Geometry check sheet. Reference: the model listing, model coordinates, mm. Face numbers are marked on the shaded views. A direction names the side the tool comes from. Give positions to 0.01 mm unless a question says otherwise; leave off trailing zeros. Loops run counter-clockwise (first coordinate to the right, second up) from the corner with the lowest first, then second, coordinate; pieces in that order, holes last. Notation, with made-up numbers: (41, -38) - (53, -38) arc R29 cw to (53, -17) - close; hole circle Ø8 at (6.25, -12.5). An arc over 180 degrees is marked (long way). Use a Markdown table: item, result. Add a question column.
1. Draft check along Z on the marked faces 3, 4, 5 and 6. Enter one of: pulls with the +Z half, pulls with the -Z half, needs draft (parallel to the pull), parting line crosses it, or undercut.
2. Cross-section at B-B on z = -15. Enter the section's corners in (x, y), and give its area (4 significant figures).
3. Set-up check for the marked faces 1 and 2: record each of +Z, -Z, +X, -X, +Y, -Y from which the full face is reachable in a straight line by a thin tool's end or side.
4. Material ranges on L1, parallel to Z at x = 25.5, y = 1; L2, parallel to Z at x = 101, y = 2.75; L3, parallel to Y at x = 8.5, z = -17.75, recorded low to high.
5. Depth check by flat-ended pin: P1, Ø2.5, axis at y = 3.5, z = -19, coming from the -X side. Enter the tip coordinate at first touch or a pass-through.
6. Cross-section at A-A on x = 101. Enter the section's corners in (y, z), and give its area (3 significant figures).
7. Cross-section at C-C on z = -6.25. Count the separate pieces of the cut face and the enclosed holes in it, and give its area (3 significant figures).
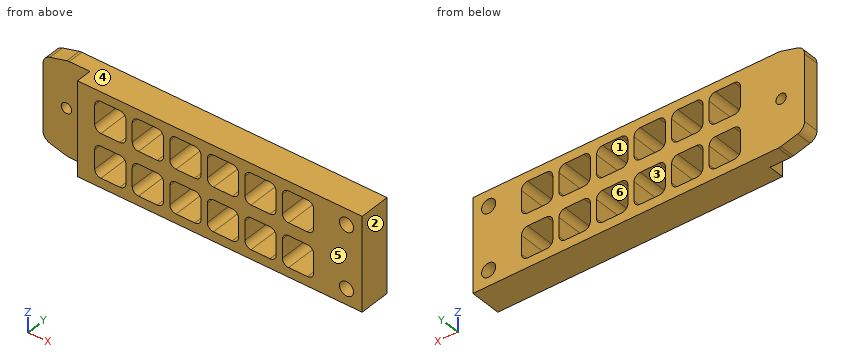
from build123d import *

# Parameters (mm, degrees)
EXTRUDE_1_DEPTH     = 10
SKETCH_4_W          = 15
SKETCH_4_H          = 30
CUT_EXTRUDE_2_DEPTH = 5
FILLET_1_R          = 3
CUT_EXTRUDE_3_DEPTH = 111.616454472
HOLE_WIZARD_M41_D   = 4.5
M4X0_71_D           = 3.3


with BuildPart() as part:
    # Эскиз1 → Бобышка-Вытянуть1 (new body)
    with BuildSketch(Plane(origin=(0, 0, 0), x_dir=(1, 0, 0), z_dir=(0, 1, 0))):
        Polygon((15, 0), (106, 0), (106, 30), (15, 30), (8, 30), (0, 27.856406461), (0, 2.143593539), (8, 0), align=None)
    extrude(amount=EXTRUDE_1_DEPTH)

    # Эскиз4 → Вырез-Вытянуть2 (cut)
    with BuildSketch(Plane.XZ):
        with Locations((7.5, -15)):
            Rectangle(SKETCH_4_W, SKETCH_4_H)
    extrude(amount=-CUT_EXTRUDE_2_DEPTH, mode=Mode.SUBTRACT)

    # Скругление1
    fillet_1_edges = [part.edges().sort_by_distance(p)[0] for p in [
        (8, 7.5, 0),
        (0, 7.5, -2.143593539),
        (0, 7.5, -27.856406461),
        (8, 7.5, -30),
    ]]
    fillet(fillet_1_edges, radius=FILLET_1_R)

    # Эскиз5 → Вырез-Вытянуть3 (cut, through all)
    with BuildSketch(Plane.XZ):
        with BuildLine():
            Line((22.5, -17), (28.5, -17))
            ThreePointArc((28.5, -17), (29.914213562, -17.585786438), (30.5, -19))
            Line((30.5, -19), (30.5, -25))
            ThreePointArc((30.5, -25), (29.914213562, -26.414213562), (28.5, -27))
            Line((28.5, -27), (22.5, -27))
            ThreePointArc((22.5, -27), (21.085786438, -26.414213562), (20.5, -25))
            Line((20.5, -25), (20.5, -19))
            ThreePointArc((20.5, -19), (21.085786438, -17.585786438), (22.5, -17))
        make_face()
        with BuildLine():
            Line((34.5, -17), (40.5, -17))
            ThreePointArc((40.5, -17), (41.914213562, -17.585786438), (42.5, -19))
            Line((42.5, -19), (42.5, -25))
            ThreePointArc((42.5, -25), (41.914213562, -26.414213562), (40.5, -27))
            Line((40.5, -27), (34.5, -27))
            ThreePointArc((34.5, -27), (33.085786438, -26.414213562), (32.5, -25))
            Line((32.5, -25), (32.5, -19))
            ThreePointArc((32.5, -19), (33.085786438, -17.585786438), (34.5, -17))
        make_face()
        with BuildLine():
            Line((46.5, -17), (52.5, -17))
            ThreePointArc((52.5, -17), (53.914213562, -17.585786438), (54.5, -19))
            Line((54.5, -19), (54.5, -25))
            ThreePointArc((54.5, -25), (53.914213562, -26.414213562), (52.5, -27))
            Line((52.5, -27), (46.5, -27))
            ThreePointArc((46.5, -27), (45.085786438, -26.414213562), (44.5, -25))
            Line((44.5, -25), (44.5, -19))
            ThreePointArc((44.5, -19), (45.085786438, -17.585786438), (46.5, -17))
        make_face()
        with BuildLine():
            Line((58.5, -17), (64.5, -17))
            ThreePointArc((64.5, -17), (65.914213562, -17.585786438), (66.5, -19))
            Line((66.5, -19), (66.5, -25))
            ThreePointArc((66.5, -25), (65.914213562, -26.414213562), (64.5, -27))
            Line((64.5, -27), (58.5, -27))
            ThreePointArc((58.5, -27), (57.085786438, -26.414213562), (56.5, -25))
            Line((56.5, -25), (56.5, -19))
            ThreePointArc((56.5, -19), (57.085786438, -17.585786438), (58.5, -17))
        make_face()
        with BuildLine():
            Line((70.5, -17), (76.5, -17))
            ThreePointArc((76.5, -17), (77.914213562, -17.585786438), (78.5, -19))
            Line((78.5, -19), (78.5, -25))
            ThreePointArc((78.5, -25), (77.914213562, -26.414213562), (76.5, -27))
            Line((76.5, -27), (70.5, -27))
            ThreePointArc((70.5, -27), (69.085786438, -26.414213562), (68.5, -25))
            Line((68.5, -25), (68.5, -19))
            ThreePointArc((68.5, -19), (69.085786438, -17.585786438), (70.5, -17))
        make_face()
        with BuildLine():
            Line((82.5, -17), (88.5, -17))
            ThreePointArc((88.5, -17), (89.914213562, -17.585786438), (90.5, -19))
            Line((90.5, -19), (90.5, -25))
            ThreePointArc((90.5, -25), (89.914213562, -26.414213562), (88.5, -27))
            Line((88.5, -27), (82.5, -27))
            ThreePointArc((82.5, -27), (81.085786438, -26.414213562), (80.5, -25))
            Line((80.5, -25), (80.5, -19))
            ThreePointArc((80.5, -19), (81.085786438, -17.585786438), (82.5, -17))
        make_face()
        with BuildLine():
            Line((90.5, -11), (90.5, -5))
            ThreePointArc((90.5, -5), (89.914213562, -3.585786438), (88.5, -3))
            Line((88.5, -3), (82.5, -3))
            ThreePointArc((82.5, -3), (81.085786438, -3.585786438), (80.5, -5))
            Line((80.5, -5), (80.5, -11))
            ThreePointArc((80.5, -11), (81.085786438, -12.414213562), (82.5, -13))
            Line((82.5, -13), (88.5, -13))
            ThreePointArc((88.5, -13), (89.914213562, -12.414213562), (90.5, -11))
        make_face()
        with BuildLine():
            Line((78.5, -11), (78.5, -5))
            ThreePointArc((78.5, -5), (77.914213562, -3.585786438), (76.5, -3))
            Line((76.5, -3), (70.5, -3))
            ThreePointArc((70.5, -3), (69.085786438, -3.585786438), (68.5, -5))
            Line((68.5, -5), (68.5, -11))
            ThreePointArc((68.5, -11), (69.085786438, -12.414213562), (70.5, -13))
            Line((70.5, -13), (76.5, -13))
            ThreePointArc((76.5, -13), (77.914213562, -12.414213562), (78.5, -11))
        make_face()
        with BuildLine():
            Line((66.5, -11), (66.5, -5))
            ThreePointArc((66.5, -5), (65.914213562, -3.585786438), (64.5, -3))
            Line((64.5, -3), (58.5, -3))
            ThreePointArc((58.5, -3), (57.085786438, -3.585786438), (56.5, -5))
            Line((56.5, -5), (56.5, -11))
            ThreePointArc((56.5, -11), (57.085786438, -12.414213562), (58.5, -13))
            Line((58.5, -13), (64.5, -13))
            ThreePointArc((64.5, -13), (65.914213562, -12.414213562), (66.5, -11))
        make_face()
        with BuildLine():
            Line((54.5, -11), (54.5, -5))
            ThreePointArc((54.5, -5), (53.914213562, -3.585786438), (52.5, -3))
            Line((52.5, -3), (46.5, -3))
            ThreePointArc((46.5, -3), (45.085786438, -3.585786438), (44.5, -5))
            Line((44.5, -5), (44.5, -11))
            ThreePointArc((44.5, -11), (45.085786438, -12.414213562), (46.5, -13))
            Line((46.5, -13), (52.5, -13))
            ThreePointArc((52.5, -13), (53.914213562, -12.414213562), (54.5, -11))
        make_face()
        with BuildLine():
            Line((42.5, -11), (42.5, -5))
            ThreePointArc((42.5, -5), (41.914213562, -3.585786438), (40.5, -3))
            Line((40.5, -3), (34.5, -3))
            ThreePointArc((34.5, -3), (33.085786438, -3.585786438), (32.5, -5))
            Line((32.5, -5), (32.5, -11))
            ThreePointArc((32.5, -11), (33.085786438, -12.414213562), (34.5, -13))
            Line((34.5, -13), (40.5, -13))
            ThreePointArc((40.5, -13), (41.914213562, -12.414213562), (42.5, -11))
        make_face()
        with BuildLine():
            Line((30.5, -11), (30.5, -5))
            ThreePointArc((30.5, -5), (29.914213562, -3.585786438), (28.5, -3))
            Line((28.5, -3), (22.5, -3))
            ThreePointArc((22.5, -3), (21.085786438, -3.585786438), (20.5, -5))
            Line((20.5, -5), (20.5, -11))
            ThreePointArc((20.5, -11), (21.085786438, -12.414213562), (22.5, -13))
            Line((22.5, -13), (28.5, -13))
            ThreePointArc((28.5, -13), (29.914213562, -12.414213562), (30.5, -11))
        make_face()
    extrude(amount=-CUT_EXTRUDE_3_DEPTH, mode=Mode.SUBTRACT)

    # Отверстие с зазором M41 (through all)
    with Locations(Plane(origin=(0, 10, 0), x_dir=(1, 0, 0), z_dir=(0, 1, 0))):
        with Locations((101, 25), (101, 5)):
            Hole(HOLE_WIZARD_M41_D / 2)

    # Отверстие обработанное метчиком M4x0.71 (through all)
    with Locations(Plane(origin=(0, 5, 0), x_dir=(-1, 0, 0), z_dir=(0, -1, 0))):
        with Locations((-7.5, 15)):
            Hole(M4X0_71_D / 2)


solid = part.part
Values found:
| question | item | result |
|---|---|---|
| 1 | face 3 | undercut |
| 1 | face 4 | pulls with the +Z half |
| 1 | face 5 | needs draft |
| 1 | face 6 | undercut |
| 2 | outline | (0, 5) - (5.85, 5) - (5.85, 10) - (0, 10) - close; (9.15, 5) - (15, 5) - (15, 0) - (106, 0) - (106, 10) - (9.15, 10) - close |
| 2 | area | 968.5 mm2 |
| 3 | face 1 | +Y, -Y |
| 3 | face 2 | +Z, -Z, +X, +Y, -Y |
| 4 | L1 | z = -30 to -27, -17 to -13, -3 to 0 |
| 4 | L2 | z = -30 to -27.25, -22.75 to -7.25, -2.75 to 0 |
| 4 | L3 | y = 5 to 10 |
| 5 | P1 | stops at x = 15 |
| 6 | outline | (0, -30) - (10, -30) - (10, -27.25) - (0, -27.25) - close; (0, -22.75) - (10, -22.75) - (10, -7.25) - (0, -7.25) - close; (0, -2.75) - (10, -2.75) - (10, 0) - (0, 0) - close |
| 6 | area | 210 mm2 |
| 7 | separate pieces | 8 |
| 7 | enclosed holes | 0 |
| 7 | area | 348 mm2 |
